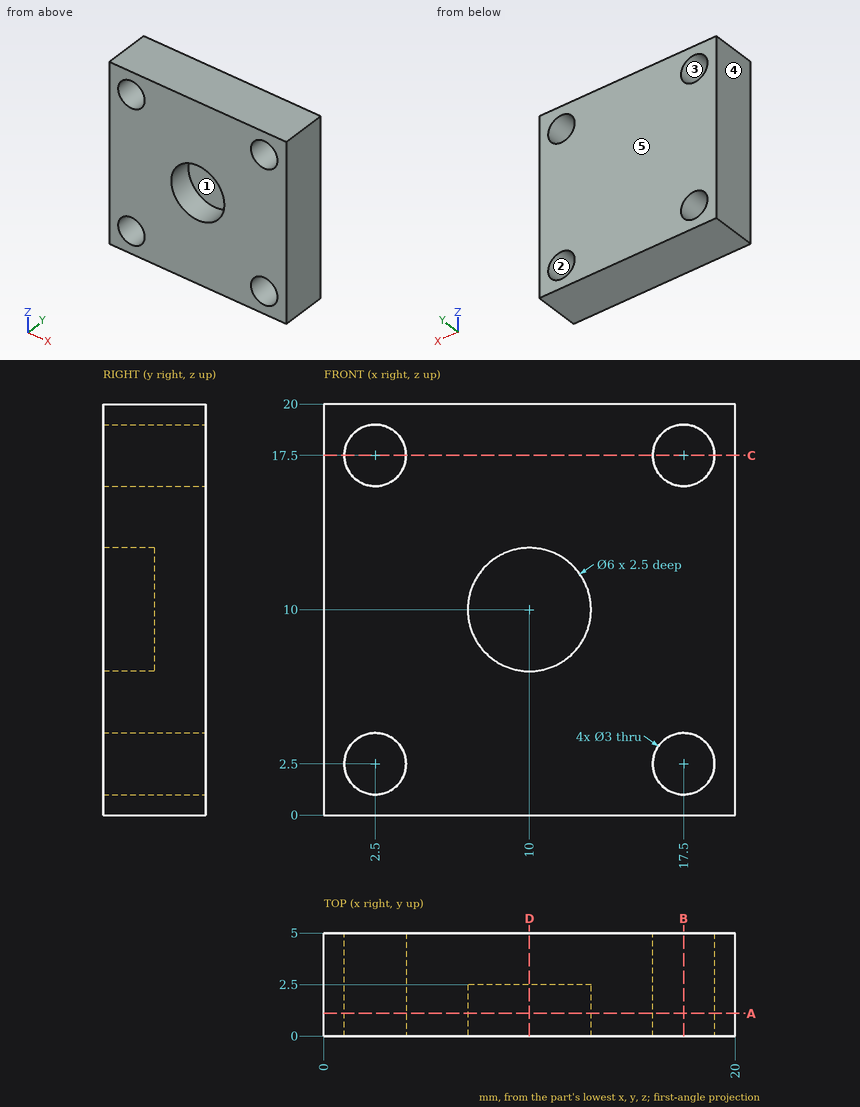
Design review of the part shown in the three views and the two pictorial views. Dimensions are in mm from the part's minimum x, y and z. A direction names the side the tool comes from. Give positions to 0.01 mm unless a question says otherwise; leave off trailing zeros. Write each loop counter-clockwise with the first axis right and the second up, starting at its lowest first coordinate (ties: lowest second). Pieces come first, ordered by that corner, then holes. Notation, with made-up numbers: M -36.75,35.25 L 20.25,35.25 A35 cw 20.25,72.25 Z; hole C 27,74 d3. An arc over 180 degrees is marked long. One line per question, with ' | ' between items. Start each with the question number.
Item 1: We need section D-D on x = 10. Write out the cut boundary in (y, z).
Item 2: For pin 1 (4 mm diameter, centred on x = 5.5, z = 16.5, fed in from -Y); pin 2 (2.5 mm diameter, centred on x = 2.5, z = 17.5, fed in from -Y), all flat-tipped, find the tip position at first contact; note any pin that passes through.
Item 3: Draft analysis for pull direction X (two halves, no side actions). For the marked faces 3, 4 and 5, state which applies: released by +X, released by -X, zero draft, split by the parting line, or undercut.
Item 4: We need section A-A on y = 1.1. Write out the cut boundary in (x, z), plus the area to 3 significant figures.
Item 5: We need section B-B on x = 17.5. Write out the cut boundary in (y, z).
Item 6: Wall thickness on line 1 (X direction, y = 3.7, z = 2.5); line 2 (Z direction, x = 2, y = 4.7): over which ranges is each line inside the solid? List them lowest first. Write a range as from..to.
Item 7: For the marked faces 1 and 2, list the 3-axis set-ups (+Z, -Z, +X, -X, +Y, -Y) from which the entire face can be reached by the end or side of a thin tool; tool diameter is ignored.
Item 8: We need section C-C on z = 17.5. Write out the cut boundary in (x, y).
Results found:
1) outline: M 0,0 L 5,0 L 5,20 L 0,20 L 0,13 L 2.5,13 L 2.5,7 L 0,7 Z
2) pin 1: stops at y = 0 | pin 2: passes through
3) face 3: undercut | face 4: released by -X | face 5: zero draft
4) outline: M 0,0 L 20,0 L 20,20 L 0,20 Z; hole C 2.5,2.5 d3; hole C 2.5,17.5 d3; hole C 10,10 d6; hole C 17.5,2.5 d3; hole C 17.5,17.5 d3 | area: 343 mm2
5) outline: M 0,0 L 5,0 L 5,1 L 0,1 Z; M 0,4 L 5,4 L 5,16 L 0,16 Z; M 0,19 L 5,19 L 5,20 L 0,20 Z
6) line 1: x = 0..1, 4..16, 19..20 | line 2: z = 0..1.09, 3.91..16.09, 18.91..20
7) face 1: -Y | face 2: +Y, -Y
8) outline: M 0,0 L 1,0 L 1,5 L 0,5 Z; M 4,0 L 16,0 L 16,5 L 4,5 Z; M 19,0 L 20,0 L 20,5 L 19,5 Z
